Work out the finished part from the listing and answer in its coordinate system (mm). A direction names the side the tool comes from. Give positions to 0.01 mm unless a question says otherwise; leave off trailing zeros. Write each loop counter-clockwise with the first axis right and the second up, starting at its lowest first coordinate (ties: lowest second). Pieces come first, ordered by that corner, then holes. Notation, with made-up numbers: (36, 15.25) - (49, 15.25) arc R29 ccw to (49, 41.25) - close; hole circle Ø9 at (-21.75, 4.25). An arc over 180 degrees is marked (long way). Write item = value, one per line.
from build123d import *

# Parameters (mm, degrees)
SKETCH1_W             = 15
SKETCH1_H             = 10
BOSS_EXTRUDE2_DEPTH   = 10
BOSS_EXTRUDE2_2_DEPTH = 10
BOSS_EXTRUDE3_DEPTH   = 10
FILLET1_R             = 0.2
FILLET2_R             = 1
FILLET3_R             = 0.5


with BuildPart() as part:
    # Sketch1 → Boss-Extrude2 (new body)
    with BuildSketch(Plane(origin=(0, 0, 0), x_dir=(1, 0, 0), z_dir=(0, 1, 0))):
        with Locations((0, 20)):
            Rectangle(SKETCH1_W, SKETCH1_H)
    extrude(amount=BOSS_EXTRUDE2_DEPTH)



with BuildPart() as body_2:
    # Sketch1 → Boss-Extrude2 2 (new body)
    with BuildSketch(Plane(origin=(0, 0, 0), x_dir=(1, 0, 0), z_dir=(0, 1, 0))):
        Rectangle(SKETCH1_W, SKETCH1_H)
    extrude(amount=BOSS_EXTRUDE2_2_DEPTH)


with BuildPart() as part_1:
    add(part.part)

    add(body_2.part)  # Boss-Extrude3 merges body 2
    # Sketch1<4> → Boss-Extrude3 (add)
    with BuildSketch(Plane(origin=(0, 0, 0), x_dir=(1, 0, 0), z_dir=(0, 1, 0))):
        Polygon((-20, 10), (0, 15), (-7.009279564, 15), (-27.009279564, 10), (-7.009279564, 5), (0, 5), align=None)
    boss_extrude3 = extrude(amount=BOSS_EXTRUDE3_DEPTH)

    # Mirror1: Boss-Extrude3 across plane
    add(boss_extrude3.mirror(Plane.ZY))

    # Fillet1
    # the kernel refuses this fillet: 0.2 mm, written as the material it adds along each edge
    with BuildSketch(Plane(origin=(7.009279564, 0, -5), x_dir=(1, 0, 0), z_dir=(0, 1, 0)), Plane(origin=(-7.009279564, 0, -15), x_dir=(-1, 0, 0), z_dir=(0, 1, 0))) as fillet1_piece_1:
        with BuildLine():
            CenterArc((0.687772533, -0.034212148), FILLET1_R, 104.036243468, 66.114258118)
            Line((0.639265408, 0.159816352), (0, 0))
            Line((0, 0), (0.490720436, 0))
        make_face()
    extrude(amount=10)
    with BuildSketch(Plane(origin=(7.009279564, 0, -15), x_dir=(1, 0, 0), z_dir=(0, 1, 0)), Plane(origin=(-7.009279564, 0, -5), x_dir=(-1, 0, 0), z_dir=(0, 1, 0))) as fillet1_piece_2:
        with BuildLine():
            CenterArc((0.687772533, 0.034212148), FILLET1_R, 189.849498414, 66.114258118)
            Line((0.639265408, -0.159816352), (0, 0))
            Line((0, 0), (0.490720436, 0))
        make_face()
    extrude(amount=10)
    with BuildSketch(Plane(origin=(0, 0, -5), x_dir=(-0.9701425001453327, 0, -0.24253562503632975), z_dir=(0, 1, 0))) as fillet1_piece_3:
        with BuildLine():
            CenterArc((FILLET1_R * 0.25, -FILLET1_R), FILLET1_R, 90, 28.072486936)
            Line((-FILLET1_R * 0.220588235294, -FILLET1_R * 0.117647058824), (0, 0))
            Line((0, 0), (FILLET1_R * 0.25, 0))
        make_face()
    extrude(amount=10)
    with BuildSketch(Plane(origin=(20, 0, -10), x_dir=(-0.9701425001453313, 0, 0.24253562503633505), z_dir=(0, 1, 0))) as fillet1_piece_4:
        with BuildLine():
            CenterArc((FILLET1_R * 4, -FILLET1_R), FILLET1_R, 90, 151.927513064)
            Line((FILLET1_R * 3.52941176471, -FILLET1_R * 1.88235294118), (0, 0))
            Line((0, 0), (FILLET1_R * 4, 0))
        make_face()
    extrude(amount=10)
    with BuildSketch(Plane(origin=(0, 0, -15), x_dir=(-0.9701425001453277, 0, 0.2425356250363498), z_dir=(0, 1, 0))) as fillet1_piece_5:
        with BuildLine():
            CenterArc((FILLET1_R * 0.25, FILLET1_R), FILLET1_R, 241.927513064, 28.072486936)
            Line((-FILLET1_R * 0.220588235294, FILLET1_R * 0.117647058824), (0, 0))
            Line((0, 0), (FILLET1_R * 0.25, 0))
        make_face()
    extrude(amount=10)
    with BuildSketch(Plane(origin=(-20, 0, -10), x_dir=(0.9701425001453319, 0, 0.24253562503633297), z_dir=(0, 1, 0))) as fillet1_piece_6:
        with BuildLine():
            CenterArc((FILLET1_R * 4, FILLET1_R), FILLET1_R, 118.072486936, 151.927513064)
            Line((FILLET1_R * 3.52941176471, FILLET1_R * 1.88235294118), (0, 0))
            Line((0, 0), (FILLET1_R * 4, 0))
        make_face()
    extrude(amount=10)

    # Fillet2
    fillet2_edges = [part_1.edges().sort_by_distance(p)[0] for p in [
        (-27.009279564, 5, -10),
        (27.009279564, 5, -10),
    ]]
    fillet(fillet2_edges, radius=FILLET2_R)

    # Fillet3
    fillet3_edges = [part_1.edges().sort_by_distance(p)[0] for p in [
        (-7.5, 5, 5),
        (7.5, 5, 5),
        (-7.5, 5, -25),
        (7.5, 5, -25),
    ]]
    fillet(fillet3_edges, radius=FILLET3_R)


solid = part_1.part
1. Find section A-A, the plane x = 3. Give the vertices of the cut face in (y, z), then the cut area to 3 significant figures.
Solution:
outline = (0, -25) - (10, -25) - (10, -14.25) - (0, -14.25) - close; (0, -5.75) - (10, -5.75) - (10, 5) - (0, 5) - close
area = 215 mm^2
2. A tool of negligible diameter and unlimited length cuts with its end or side. For faces 1 (the flat face through (7.5, 5, 0)), 2 (the flat face through (-9.77, 4.93, -12.557)), 3 (the flat face through (-7.5, 5, -20)), 4 (the flat face through (7.5, 5, -20)), 5 (the flat face through (-7.5, 5, 0)), from which of +Z, -Z, +X, -X, +Y, -Y can it reach the whole face along a straight path? Write none if from no direction.
Solution:
face_1 = +Z, +X, +Y, -Y
face_2 = +Y, -Y
face_3 = -Z, -X, +Y, -Y
face_4 = -Z, +X, +Y, -Y
face_5 = +Z, -X, +Y, -Y
3. Given pin 1 (5 mm diameter, centred on y = 3, z = -2, fed in from +X); pin 2 (4 mm diameter, centred on y = 7, z = -7.5, fed in from -X); pin 3 (3 mm diameter, centred on y = 3, z = 0.5, fed in from -X), each flat-ended and moving along its own axis, determine where each tip first touches the part or whether it passes through.
Solution:
pin_1 = 7.5
pin_2 = -23.75
pin_3 = -7.5
4. Find section D-D, the plane z = -17. Give the vertices of the cut face in (x, y), then the cut area to 3 significant figures.
Solution:
outline = (-7.5, 0) - (7.5, 0) - (7.5, 10) - (-7.5, 10) - close
area = 150 mm^2
5. For a pull along X with two mould halves and no side action, classify faces 6 (the flat face through (-9.502, 4.93, -7.375)), 7 (the flat face through (-15.497, 4.93, -7.122)), 8 (the flat face through (5, 0, -14)) as pulls with the +X half, pulls with the -X half, needs draft (parallel to the pull), parting line crosses it, or undercut.
Solution:
face_6 = undercut
face_7 = pulls with the -X half
face_8 = needs draft
6. Straight lines are drawn through the part: line 1 (X direction, y = 1.25, z = -10); line 2 (X direction, y = 4.5, z = -3.5); line 3 (Z direction, x = 2, y = 4.5). For each, find the intervals that lie inside material, in ascending order.
Solution:
line_1 = -23.89 to -19.38, 19.38 to 23.89
line_2 = -7.5 to 7.5
line_3 = -25 to -14.5, -5.5 to 5
7. Find section C-C, the plane z = -13. Give the vertices of the cut face in (x, y), then the cut area to 3 significant figures.
Solution:
outline = (-15.01, 0) - (-8, 0) - (-8, 10) - (-15.01, 10) - close; (8, 0) - (15.01, 0) - (15.01, 10) - (8, 10) - close
area = 140 mm^2
8. Find section B-B, the plane y = 7. Give the vertices of the cut face in (x, z).
Solution:
outline = (-23.13, -10.97) - (-7.65, -14.84) arc R0.2 cw to (-7.5, -15) - (-7.5, -24.5) arc R0.5 ccw to (-7, -25) - (7, -25) arc R0.5 ccw to (7.5, -24.5) - (7.5, -15) arc R0.2 cw to (7.65, -14.84) - (23.13, -10.97) arc R1 ccw to (23.13, -9.03) - (7.65, -5.16) arc R0.2 cw to (7.5, -5) - (7.5, 4.5) arc R0.5 ccw to (7, 5) - (-7, 5) arc R0.5 ccw to (-7.5, 4.5) - (-7.5, -5) arc R0.2 cw to (-7.65, -5.16) - (-23.13, -9.03) arc R1 ccw to start; hole (-19.22, -10.19) - (-0.05, -14.99) arc R0.2 ccw to (0.05, -14.99) - (19.22, -10.19) arc R0.2 ccw to (19.22, -9.81) - (0.05, -5.01) arc R0.2 ccw to (-0.05, -5.01) - (-19.22, -9.81) arc R0.2 ccw to start
